Geometry: final body of the model. Coordinates: model frame, mm. Give positions to 0.01 mm unless a question says otherwise; leave off trailing zeros. Loops run counter-clockwise (first coordinate to the right, second up) from the corner with the lowest first, then second, coordinate; pieces in that order, holes last.
from build123d import *

# Parameters (mm, degrees)
BOSS_EXTRUDE1_DEPTH = 3.175


with BuildPart() as part:
    # Sketch1 → Boss-Extrude1 (new body)
    with BuildSketch(Plane.XY):
        Polygon((31, 123.65), (31, 126.825), (41, 126.825), (41, 123.65), (51, 123.65), (51, 126.825), (61, 126.825), (61, 123.65), (71, 123.65), (71, 126.825), (81, 126.825), (81, 123.65), (91, 123.65), (91, 126.825), (101, 126.825), (101, 123.65), (111, 123.65), (111, 126.825), (121, 126.825), (121, 123.65), (131, 123.65), (131, 126.825), (141, 126.825), (141, 123.65), (151, 123.65), (151, 126.825), (161, 126.825), (161, 123.65), (171, 123.65), (171, 126.825), (181, 126.825), (181, 123.65), (191, 123.65), (191, 126.825), (201, 126.825), (201, 123.65), (211, 123.65), (211, 126.825), (221, 126.825), (221, 123.65), (231, 123.65), (231, 126.825), (241, 126.825), (241, 123.65), (252, 123.65), (252, 116.825), (255.175, 116.825), (255.175, 106.825), (252, 106.825), (252, 96.825), (255.175, 96.825), (255.175, 86.825), (252, 86.825), (252, 36.825), (255.175, 36.825), (255.175, 26.825), (252, 26.825), (252, 16.825), (255.175, 16.825), (255.175, 6.825), (252, 6.825), (252, 0), (241, 0), (241, -3.175), (231, -3.175), (231, 0), (221, 0), (221, -3.175), (211, -3.175), (211, 0), (201, 0), (201, -3.175), (191, -3.175), (191, 0), (181, 0), (181, -3.175), (171, -3.175), (171, 0), (161, 0), (161, -3.175), (151, -3.175), (151, 0), (141, 0), (141, -3.175), (131, -3.175), (131, 0), (121, 0), (121, -3.175), (111, -3.175), (111, 0), (101, 0), (101, -3.175), (91, -3.175), (91, 0), (81, 0), (81, -3.175), (71, -3.175), (71, 0), (61, 0), (61, -3.175), (51, -3.175), (51, 0), (41, 0), (41, -3.175), (31, -3.175), (31, 0), (21, 0), (21, -3.175), (11, -3.175), (11, 0), (0, 0), (0, 6.825), (-3.175, 6.825), (-3.175, 16.825), (0, 16.825), (0, 26.825), (-3.175, 26.825), (-3.175, 36.825), (0, 36.825), (0, 86.825), (-3.175, 86.825), (-3.175, 96.825), (0, 96.825), (0, 106.825), (-3.175, 106.825), (-3.175, 116.825), (0, 116.825), (0, 123.65), (11, 123.65), (11, 126.825), (21, 126.825), (21, 123.65), align=None)
    extrude(amount=BOSS_EXTRUDE1_DEPTH)


solid = part.part
Item 1: Pin query (flat end, axial travel): pin 1 (1.5 mm diameter, centred on x = 208.5, y = 40, fed in from -Z); pin 2 (1 mm diameter, centred on y = 119.5, z = 2, fed in from -X); pin 3 (1 mm diameter, centred on y = -1, z = 1, fed in from -X); pin 4 (1.6 mm diameter, centred on x = 253, z = 2, fed in from -Y) (3 decimals). Return the tip coordinate at first contact, or that it passes through.
Values follow:
pin 1: stops at z = 0
pin 2: stops at x = 0
pin 3: stops at x = 11
pin 4: stops at y = 6.825
Item 2: Section query A-A on y = 84.5. Return loops of the section in (x, z) (3 decimals).
Values follow:
outline: (0, 0) - (252, 0) - (252, 3.175) - (0, 3.175) - close
Item 3: Ray query, probe 1 along X at (y, z) = (83, 0.6); probe 2 along Y at (x, z) = (10, 1.3). Return the intervals inside material, ascending.
Values follow:
probe 1: x = 0 to 252
probe 2: y = 0 to 123.65
Item 4: Section query B-B on x = 124. Return loops of the section in (y, z) (3 decimals), plus the area to 3 significant figures.
Values follow:
outline: (0, 0) - (123.65, 0) - (123.65, 3.175) - (0, 3.175) - close
area: 393 mm2
